```python
from build123d import *

# Parameters (mm, degrees)
REVOLUCI_N1_ANGLE       = 180
CORTAR_EXTRUIR1_DEPTH   = 17
CORTAR_EXTRUIR2_START   = -5.65
CORTAR_EXTRUIR2_DEPTH   = 5.65
CORTAR_EXTRUIR3_START   = -23
CROQUIS4_W              = 20.036929734
CROQUIS4_H              = 3.3102989
CORTAR_EXTRUIR3_DEPTH   = 23
CROQUIS5_W              = 1
CROQUIS5_H              = 4
CORTAR_EXTRUIR4_DEPTH   = 3
CROQUIS6_W              = 10
CROQUIS6_H              = 4
SALIENTE_EXTRUIR1_DEPTH = 3


with BuildPart() as part:
    # Croquis1 → Revolución1 (revolve)
    with BuildSketch(Plane.XY):
        Polygon((-91.628819856, 0), (-106.128819856, 0), (-106.128819856, 23), (-91.378819856, 23), (-91.378819856, 20.6), (-97.878819856, 20.6), (-97.878819856, 19.35), (-91.378819856, 19.35), (-91.378819856, 17.35), (-103.128819856, 17.35), (-103.128819856, 15.35), (-91.628819856, 15.35), (-91.628819856, 9.003019764), (-103.378819856, 9.003019764), (-103.378819856, 7.703019764), (-91.628819856, 7.703019764), (-91.628819856, 4.303019764), (-103.378819856, 4.303019764), (-103.378819856, 3.003019764), (-91.628819856, 3.003019764), align=None)
    revolve(axis=Axis((-91.378819856, 17.35, 0), (0, -1, 0)), revolution_arc=REVOLUCI_N1_ANGLE)

    # Croquis2 → Cortar-Extruir1 (cut)
    with BuildSketch(Plane.XZ):
        with BuildLine():
            Line((-100.628819856, 0), (-81.628819856, 0))
            ThreePointArc((-81.628819856, 0), (-91.128819856, -9.5), (-100.628819856, 0))
        make_face()
    extrude(amount=-CORTAR_EXTRUIR1_DEPTH, mode=Mode.SUBTRACT)

    # Croquis3 → Cortar-Extruir2 (cut)
    with BuildSketch(Plane(origin=(0, 23, 0), x_dir=(1, 0, 0), z_dir=(0, 1, 0)).offset(CORTAR_EXTRUIR2_START)):
        with BuildLine():
            Line((-86.628819856, 0), (-95.628819856, 0))
            ThreePointArc((-95.628819856, 0), (-91.128819856, 4.5), (-86.628819856, 0))
        make_face()
    extrude(amount=CORTAR_EXTRUIR2_DEPTH, mode=Mode.SUBTRACT)

    # Croquis4 → Cortar-Extruir3 (cut)
    with BuildSketch(Plane.XZ.offset(CORTAR_EXTRUIR3_START)):
        with Locations((-91.493585316, -13.15514945)):
            Rectangle(CROQUIS4_W, CROQUIS4_H)
    extrude(amount=CORTAR_EXTRUIR3_DEPTH, mode=Mode.SUBTRACT)

    # Croquis5 → Cortar-Extruir4 (cut)
    with BuildSketch(Plane.XY):
        with Locations((-105.628819856, 12)):
            Rectangle(CROQUIS5_W, CROQUIS5_H)
        with Locations((-77.128819856, 12)):
            Rectangle(CROQUIS5_W, CROQUIS5_H)
    extrude(amount=-CORTAR_EXTRUIR4_DEPTH, mode=Mode.SUBTRACT)

    # Croquis6 → Saliente-Extruir1 (add)
    with BuildSketch(Plane.XY):
        with Locations((-110.128819856, 12)):
            Rectangle(CROQUIS6_W, CROQUIS6_H)
        with Locations((-72.628819856, 12)):
            Rectangle(CROQUIS6_W, CROQUIS6_H)
    extrude(amount=-SALIENTE_EXTRUIR1_DEPTH)


solid = part.part
```
Build history of the part. All positions in model axes, mm. A direction names the side the tool comes from. Round coordinates to 2 decimals unless told otherwise and drop trailing zeros. Order: outer loops, then holes, each group sorted by start corner. A loop starts at its lowest first (then second) coordinate and runs counter-clockwise, first axis right, second up. Notation, with made-up numbers: (-31, 56) - (12, 56) arc R9 ccw to (12, 66) - close; hole circle Ø1 at (5.5, 71.5). An arc over 180 degrees is marked (long way). Use a Markdown table: item, result.
1) Saw through at D-D on y = 4.75. Write the cut outline in (x, z).
Recorded:
| item | result |
|---|---|
| outline | (-106.13, 0) arc R14.75 ccw to (-100.62, -11.5) - (-82.14, -11.5) arc R14.75 ccw to (-76.63, 0) - (-81.63, 0) arc R9.5 cw to (-100.63, 0) - close |
2) Saw through at B-B on z = -8.75. Write the cut outline in (x, y).
Recorded:
| item | result |
|---|---|
| outline | (-103.25, 0) - (-94.83, 0) - (-94.83, 3) - (-99.59, 3) - (-99.59, 4.3) - (-94.83, 4.3) - (-94.83, 7.7) - (-99.59, 7.7) - (-99.59, 9) - (-94.83, 9) - (-94.83, 15.35) - (-99.22, 15.35) - (-99.22, 17.35) - (-83.54, 17.35) - (-83.54, 15.35) - (-87.43, 15.35) - (-87.43, 9) - (-83.17, 9) - (-83.17, 7.7) - (-87.43, 7.7) - (-87.43, 4.3) - (-83.17, 4.3) - (-83.17, 3) - (-87.43, 3) - (-87.43, 0) - (-79.5, 0) - (-79.5, 23) - (-103.25, 23) - close |
3) Pull direction X, two halves, no side cores. Call faces 1 (the face through (-91, 3.003, -10)), 2 (the face through (-115.129, 12, -1)), 3 (the face through (-72, 14, -1)): pulls with the +X half, pulls with the -X half, needs draft (parallel to the pull), parting line crosses it, or undercut.
Recorded:
| item | result |
|---|---|
| face 1 | undercut |
| face 2 | pulls with the -X half |
| face 3 | needs draft |
4) Tool access for faces 4 (the face through (-91, 20.6, -5)), 5 (the face through (-90.92, 12.132, -9.498)), 6 (the face through (-92, 0, -10)): list every direction of +Z, -Z, +X, -X, +Y, -Y with a clear straight run to the whole face (end or side of a thin tool).
Recorded:
| item | result |
|---|---|
| face 4 | +Z |
| face 5 | +Z, -Y |
| face 6 | +Z, -Z, +X, -X, -Y |
5) Flat gauge pins, fed straight in: pin 1 Ø3 at (x, y) = (-73.5, 11.5) entering from -Z; pin 2 Ø3.5 at (x, z) = (-112, -2) entering from +Y; pin 3 Ø2 at (y, z) = (18, -3) entering from -X. Where does each tip first touch, or does it go through?
Recorded:
| item | result |
|---|---|
| pin 1 | stops at z = -3 |
| pin 2 | stops at y = 14 |
| pin 3 | stops at x = -105.99 |
6) Saw through at C-C on x = -107. Write the cut outline in (y, z), and give its area (3 significant figures).
Recorded:
| item | result |
|---|---|
| outline | (10, -3) - (14, -3) - (14, 0) - (10, 0) - close |
| area | 12.0 mm² |
7) Saw through at A-A on y = 10.5. Write the cut outline in (x, z), and give its area (3 significant figures).
Recorded:
| item | result |
|---|---|
| outline | (-115.13, -3) - (-105.82, -3) arc R14.75 ccw to (-100.62, -11.5) - (-82.14, -11.5) arc R14.75 ccw to (-76.94, -3) - (-67.63, -3) - (-67.63, 0) - (-81.63, 0) arc R9.5 cw to (-100.63, 0) - (-115.13, 0) - close |
| area | 214 mm² |
8) Wall check: L1, parallel to Y at x = -83.5, z = -6; L2, parallel to Y at x = -95.5, z = -4; L3, parallel to Y at x = -102.5, z = -4. Give the ranges that are in metal, low to high.
Recorded:
| item | result |
|---|---|
| L1 | y = 0 to 3, 4.3 to 7.7, 9 to 15.35, 17.35 to 23 |
| L2 | y = 17.35 to 19.35, 20.6 to 23 |
| L3 | y = 0 to 3, 4.3 to 7.7, 9 to 23 |
